Drawing for the job (mm, zero at the part's lowest x, y, z). A direction names the side the tool comes from. Give positions to 0.01 mm unless a question says otherwise; leave off trailing zeros. Order: outer loops, then holes, each group sorted by start corner. A loop starts at its lowest first (then second) coordinate and runs counter-clockwise, first axis right, second up. Notation, with made-up numbers: M 61,-12 L 71,-12 A25 cw 71,14 Z; hole C 89.5,68.25 d5. An arc over 180 degrees is marked long. One line per item, written item: value.
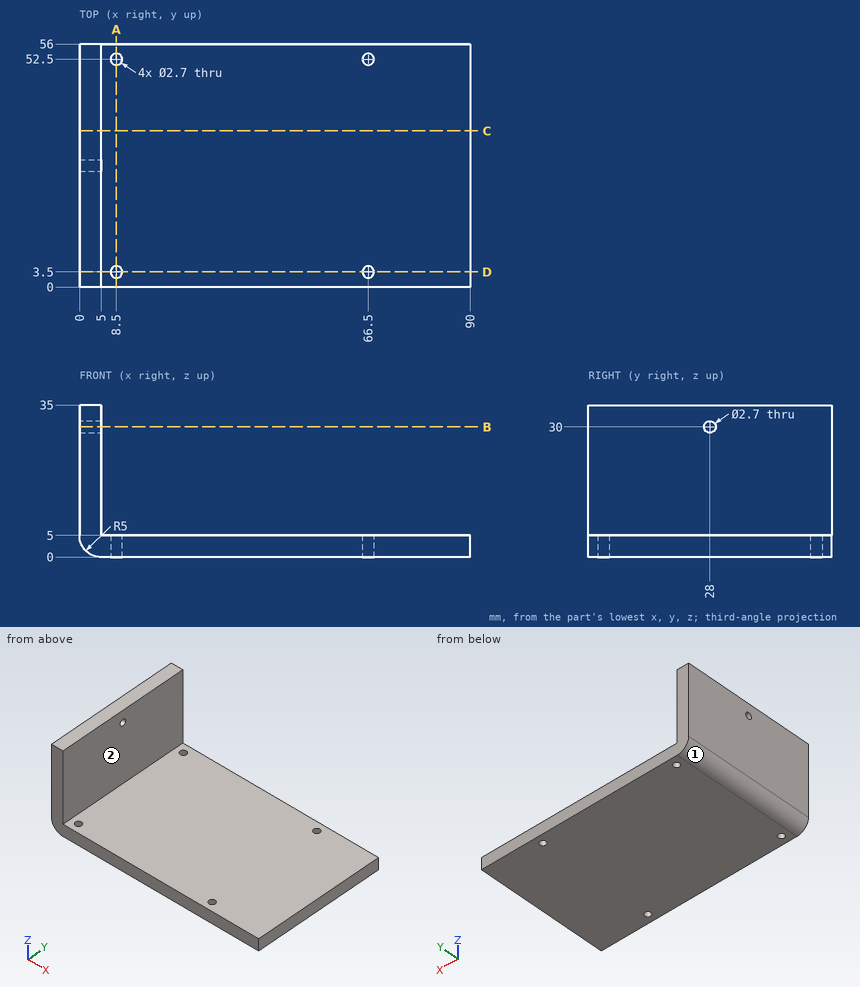
1) Pin check, flat tips, straight feed: pin 1 (1 mm diameter, centred on x = 74, y = 16, fed in from +Z); pin 2 (8 mm diameter, centred on y = 32, z = 28, fed in from +X). Stop position of each tip, or through.
Check values:
pin 1: z = 5
pin 2: x = 5
2) Saw through at D-D, the plane y = 3.5. Write the cut outline in (x, z), then the cut area to 3 significant figures.
Check values:
outline: M 0,5 A5 ccw 5,0 L 7.15,0 L 7.15,5 L 5,5 L 5,35 L 0,35 Z; M 9.85,0 L 65.15,0 L 65.15,5 L 9.85,5 Z; M 67.85,0 L 90,0 L 90,5 L 67.85,5 Z
area: 568 mm^2
3) Saw through at C-C, the plane y = 36. Write the cut outline in (x, z), then the cut area to 3 significant figures.
Check values:
outline: M 0,5 A5 ccw 5,0 L 90,0 L 90,5 L 5,5 L 5,35 L 0,35 Z
area: 595 mm^2
4) Saw through at B-B, the plane z = 30. Write the cut outline in (x, y), then the cut area to 4 significant figures.
Check values:
outline: M 0,0 L 5,0 L 5,26.65 L 0,26.65 Z; M 0,29.35 L 5,29.35 L 5,56 L 0,56 Z
area: 266.5 mm^2
5) Tool access for the marked faces 1 and 2: list every direction of +Z, -Z, +X, -X, +Y, -Y with a clear straight run to the whole face (end or side of a thin tool).
Check values:
face 1: -Z, -X, +Y, -Y
face 2: +Z, +X, +Y, -Y
6) Drill centre lines: probe 1 along Y at (x, z) = (66.5, 3.4); probe 2 along X at (y, z) = (5, 8). Where is each one in solid material? Low to high. Write a range as from..to.
Check values:
probe 1: 0..2.15, 4.85..51.15, 53.85..56
probe 2: 0..5
7) Saw through at A-A, the plane x = 8.5. Write the cut outline in (y, z).
Check values:
outline: M 0,0 L 2.15,0 L 2.15,5 L 0,5 Z; M 4.85,0 L 51.15,0 L 51.15,5 L 4.85,5 Z; M 53.85,0 L 56,0 L 56,5 L 53.85,5 Z
